Here's how the part is built. I have some questions about the finished solid (model axes, mm). Face numbers are marked on the shaded views. A direction names the side the tool comes from. Give positions to 0.01 mm unless a question says otherwise; leave off trailing zeros. Loops run counter-clockwise (first coordinate to the right, second up) from the corner with the lowest first, then second, coordinate; pieces in that order, holes last.
Q1. If we section it at A-A (x = -37): Please give me the cut outline in (y, z), plus the area to 3 significant figures.
Q2. If we section it at B-B (y = -391.5): Please give me the cut outline in (x, z).
Q3. Will these pins go through, and if not, where does the flat tip stop? P1, Ø4.5, axis at x = -196.06, y = 148.51, coming from the +Z side; P2, Ø4, axis at x = -177.5, y = -655, coming from the +Z side; P3, Ø2, axis at y = 85, z = 12.5, coming from the -X side.
Q4. If we section it at C-C (y = 32): Please give me the cut outline in (x, z), plus the area to 3 significant figures.
Q5. For the marked faces 1 and 2, which set-ups out of +Z, -Z, +X, -X, +Y, -Y let a thin tool reach every point of the face, with its end or its side?
Q6. I need wall thicknesses on line 1 (Z direction, x = -113, y = 164.5). Which ranges of the line are inside material? Lowest first, please.
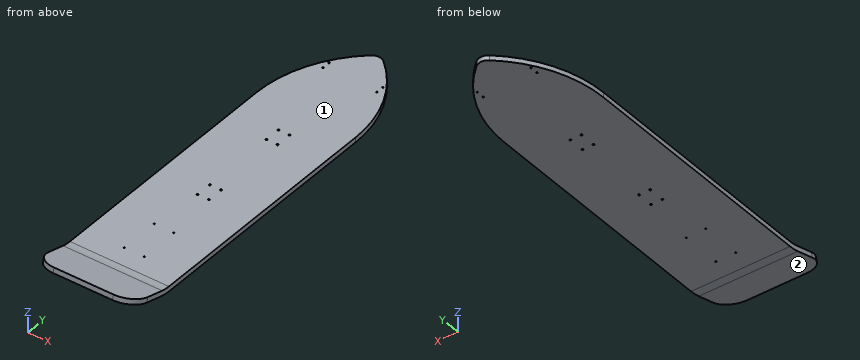
from build123d import *

# Parameters (mm, degrees)
F1_DEPTH = 12.7
F2_R     = 25.4
F4_DEPTH = 254
F5_R     = 50.8
F6_R     = 2.15265
F6_R_2   = 1.5875
F6_R_3   = 1.7272
F7_DEPTH = 12.7


with BuildPart() as f1:
    # F0 (on Top) → F1 (new body)
    with BuildSketch(Plane.XY):
        with BuildLine():
            Line((-254, -635), (0, -635))
            Line((0, -635), (0, 0))
            ThreePointArc((0, 0), (-33.5193668575, 141.9903165712), (-127, 254))
            ThreePointArc((-127, 254), (-220.4806331425, 141.9903165712), (-254, 0))
            Line((-254, 0), (-254, -635))
        make_face()
    extrude(amount=F1_DEPTH)

    # F2
    f2_edges = [f1.edges().sort_by_distance(p)[0] for p in [
        (-127, 254, 6.35),
    ]]
    fillet(f2_edges, radius=F2_R)

    # F3 (on face) → F4 (join, through all)
    with BuildSketch(Plane(origin=(-254, 0, 0), x_dir=(0, -1, 0), z_dir=(-1, 0, 0))):
        with BuildLine():
            ThreePointArc((658.0090131096, 15.7291940429), (646.6037784884, 13.4605518239), (635, 12.7))
            Line((635, 12.7), (635, 0))
            ThreePointArc((635, 0), (648.2614611296, 0.8692020844), (661.2960149824, 3.461936049))
            Line((661.2960149824, 3.461936049), (759.4340789334, 29.7579510314))
            Line((759.4340789334, 29.7579510314), (756.1470770606, 42.0252090253))
            Line((756.1470770606, 42.0252090253), (658.0090131096, 15.7291940429))
        make_face()
    extrude(amount=-F4_DEPTH)

    # F5
    f5_edges = [f1.edges().sort_by_distance(p)[0] for p in [
        (0, -757.790578, 35.89158),
        (-254, -757.790578, 35.89158),
    ]]
    fillet(f5_edges, radius=F5_R)

    # F6 (on face) → F7 (cut, through all)
    with BuildSketch(Plane.XY.offset(12.7)):
        with Locations((-112.7125, -308.7116213322)):
            Circle(F6_R)
        with Locations((-141.2875, -308.7116213322)):
            Circle(F6_R)
        with Locations((-101.6, -584.7842693329)):
            Circle(F6_R_2)
        with Locations((-152.4, -584.7842693329)):
            Circle(F6_R_2)
        with Locations((-152.4, -483.1842693329)):
            Circle(F6_R_2)
        with Locations((-101.6, -483.1842693329)):
            Circle(F6_R_2)
        with Locations((-141.2875, -75.0787870646)):
            Circle(F6_R)
        with Locations((-112.7125, -75.0787870646)):
            Circle(F6_R)
        with Locations((-112.7125, -116.3537870646)):
            Circle(F6_R)
        with Locations((-141.2875, -116.3537870646)):
            Circle(F6_R)
        with Locations((-141.2875, -349.9866213322)):
            Circle(F6_R)
        with Locations((-112.7125, -349.9866213322)):
            Circle(F6_R)
        with Locations((-57.94375, 169.1481069684)):
            Circle(F6_R_3)
        with Locations((-57.94375, 148.5106069684)):
            Circle(F6_R_3)
        with Locations((-196.05625, 148.5106069684)):
            Circle(F6_R_3)
        with Locations((-196.05625, 169.1481069684)):
            Circle(F6_R_3)
    extrude(amount=-F7_DEPTH, mode=Mode.SUBTRACT)


solid = f1.part
Check sheet entries:
1. outline: (-757.59, 29.26) - (-661.3, 3.46) arc R101.6 ccw to (-635, 0) - (148.75, 0) - (148.75, 12.7) - (-635, 12.7) arc R88.9 cw to (-658.01, 15.73) - (-754.3, 41.53) - close
1. area: 11,500 mm2
2. outline: (-254, 0) - (0, 0) - (0, 12.7) - (-254, 12.7) - close
3. P1: stops at z = 12.7
3. P2: stops at z = 15.47
3. P3: stops at x = -242.69
4. outline: (-252.38, 0) - (-1.62, 0) - (-1.62, 12.7) - (-252.38, 12.7) - close
4. area: 3,180 mm2
5. face 1: +Z, +X, -X, +Y
5. face 2: -Z, +X, -X, -Y
6. line 1: z = 0 to 12.7
